Part model, mm, in its own coordinate system. A direction names the side the tool comes from. Coordinates: 2 decimals unless noted, no trailing zeros. Order: outer loops, then holes, each group sorted by start corner. A loop starts at its lowest first (then second) coordinate and runs counter-clockwise, first axis right, second up. Notation, with made-up numbers: (-4.75, 66.25) - (1.25, 66.25) arc R17 ccw to (1.25, 88.25) - close; hole circle Ø7 at (23.25, 81.5). An arc over 180 degrees is marked (long way). Use a Markdown table: item, result. Add a question column.
1) Saw through at A-A on x = 0. List the corners of the cut face in (y, z), then the cut area to 3 significant figures.
2) Drop flat-ended pins along their axis: P1, Ø2, axis at x = 23.241, z = 0, coming from the -Y side; P2, Ø3.5, axis at x = 0, z = 0, coming from the +Y side; P3, Ø1.5, axis at y = 3, z = -2.5, coming from the -X side; P4, Ø2, axis at x = 11.5, y = 3.5, coming from the -Z side. Give the stop position or say it passes through.
3) Saw through at B-B on z = 0. List the corners of the cut face in (x, y) (3 decimals).
4) Two-plate mould, pull along X, no slides. Class faces 1 (the face through (0, 0, 3)), 2 (the face through (20.836, 3.549, 0.41)), 3 (the face through (3.35, 1.5, 0.74)), 4 (the face through (22.5, 3.55, -0.17)): +X half, -X half, draft (parallel to the pull), parting line (faces both ways), or undercut.
5) Saw through at D-D on y = 1.4. List the corners of the cut face in (x, z).
6) Saw through at C-C on y = 3.7. List the corners of the cut face in (x, z) (3 decimals), then the cut area to 3 significant figures.
7) Tool access for faces 5 (the face through (11, 4.064, 0)), 6 (the face through (2.728, 1.503, 0.606)): list every direction of +Z, -Z, +X, -X, +Y, -Y with a clear straight run to the whole face (end or side of a thin tool).
8) Wall check: L1, parallel to X at y = 3.95, z = 0.5; L2, parallel to Y at x = 22, z = -2; L3, parallel to Z at x = -1, y = 3.45. Give the ranges that are in metal, low to high. Write a range as [from, to].
```python
from build123d import *

# Parameters (mm, degrees)
SKETCH5_R           = 3.429
SKETCH5_R_2         = 2.794
BOSS_EXTRUDE3_DEPTH = 3.048
SKETCH6_R           = 0.762
SKETCH6_R_2         = 1.27
BOSS_EXTRUDE4_DEPTH = 1.016


with BuildPart() as part:
    # Sketch5 → Boss-Extrude3 (new body)
    with BuildSketch(Plane(origin=(0, 0, 0), x_dir=(1, 0, 0), z_dir=(0, 1, 0))):
        with Locations(Location((0, 0, 0), (0, 0, 90))):
            Circle(SKETCH5_R)
        with Locations(Location((0, 0, 0), (0, 0, 90))):
            Circle(SKETCH5_R_2, mode=Mode.SUBTRACT)
    extrude(amount=BOSS_EXTRUDE3_DEPTH)

    # Sketch6 → Boss-Extrude4 (add)
    with BuildSketch(Plane(origin=(0, 3.048, 0), x_dir=(1, 0, 0), z_dir=(0, 1, 0))):
        with BuildLine():
            ThreePointArc((0.275010076, 4.054684385), (-4.064, 0), (0.275010076, -4.054684385))
            Line((0.275010076, -4.054684385), (23.241, -2.497009847))
            ThreePointArc((23.241, -2.497009847), (25.738009847, 0), (23.241, 2.497009847))
            Line((23.241, 2.497009847), (0.275010076, 4.054684385))
        make_face()
        with Locations(Location((20.193, 0, 0), (0, 0, 270))):
            Circle(SKETCH6_R, mode=Mode.SUBTRACT)
        with Locations(Location((0, 0, 0), (0, 0, 270))):
            Circle(SKETCH6_R_2, mode=Mode.SUBTRACT)
        with Locations(Location((17.145, 0, 0), (0, 0, 270))):
            Circle(SKETCH6_R, mode=Mode.SUBTRACT)
        with Locations(Location((23.241, 0, 0), (0, 0, 270))):
            Circle(SKETCH6_R, mode=Mode.SUBTRACT)
    extrude(amount=BOSS_EXTRUDE4_DEPTH)


solid = part.part
```
Results are:
| question | item | result |
|---|---|---|
| 1 | outline | (0, -3.43) - (3.05, -3.43) - (3.05, -4.06) - (4.06, -4.06) - (4.06, -1.27) - (3.05, -1.27) - (3.05, -2.79) - (0, -2.79) - close; (0, 2.79) - (3.05, 2.79) - (3.05, 1.27) - (4.06, 1.27) - (4.06, 4.06) - (3.05, 4.06) - (3.05, 3.43) - (0, 3.43) - close |
| 1 | area | 9.55 mm2 |
| 2 | P1 | y = 3.05 |
| 2 | P2 | y = 4.06 |
| 2 | P3 | x = -3.67 |
| 2 | P4 | z = -3.36 |
| 3 | outline | (-4.064, 3.048) - (-3.429, 3.048) - (-3.429, 0) - (-2.794, 0) - (-2.794, 3.048) - (-1.27, 3.048) - (-1.27, 4.064) - (-4.064, 4.064) - close; (1.27, 3.048) - (2.794, 3.048) - (2.794, 0) - (3.429, 0) - (3.429, 3.048) - (16.383, 3.048) - (16.383, 4.064) - (1.27, 4.064) - close; (17.907, 3.048) - (19.431, 3.048) - (19.431, 4.064) - (17.907, 4.064) - close; (20.955, 3.048) - (22.479, 3.048) - (22.479, 4.064) - (20.955, 4.064) - close; (24.003, 3.048) - (25.738, 3.048) - (25.738, 4.064) - (24.003, 4.064) - close |
| 4 | face 1 | draft |
| 4 | face 2 | undercut |
| 4 | face 3 | parting line |
| 4 | face 4 | undercut |
| 5 | outline | circle Ø6.86 at (0, 0); hole circle Ø5.59 at (0, 0) |
| 6 | outline | (0.275, -4.055) - (23.241, -2.497) arc R2.497 ccw to (23.241, 2.497) - (0.275, 4.055) arc R4.064 ccw (long way) to start; hole circle Ø2.54 at (0, 0); hole circle Ø1.524 at (17.145, 0); hole circle Ø1.524 at (20.193, 0); hole circle Ø1.524 at (23.241, 0) |
| 6 | area | 178 mm2 |
| 7 | face 5 | +Z, -Z, +X, -X, +Y |
| 7 | face 6 | -Y |
| 8 | L1 | [-4.03, -1.17], [1.17, 16.57], [17.72, 19.62], [20.77, 22.67], [23.82, 25.69] |
| 8 | L2 | [3.05, 4.06] |
| 8 | L3 | [-3.94, -0.78], [0.78, 3.94] |
